from build123d import *

# Parameters (mm, degrees)
SKETCH1_W                                    = 150
SKETCH1_H                                    = 100
EXTRUDE1_DEPTH                               = 20
EXTRUDE2_DEPTH                               = 15
FILLET1_R                                    = 20
CBORE_FOR_M8_HEX_SOCKET_HEAD_CAP_SCR_2_COUNT = 2
CBORE_FOR_M8_HEX_SOCKET_HEAD_CAP_SCR_2_PITCH = 125.099960032
M8_TAPPED_HOLE1_AT_2_COUNT                   = 2
M8_TAPPED_HOLE1_AT_2_PITCH                   = 45
F_8_0_8_DIAMETER_HOLE1_AT_2_COUNT            = 2
F_8_0_8_DIAMETER_HOLE1_AT_2_PITCH            = 70
EXTRUDE3_DEPTH                               = 7
FILLET2_R                                    = 3
FILLET3_R                                    = 10
CHAMFER1_SIZE                                = 0.5
CHAMFER2_SIZE                                = 2
FILLET4_R                                    = 1
SKETCH10_W                                   = 30
SKETCH10_H                                   = 32
EXTRUDE4_DEPTH                               = 5
FILLET5_R                                    = 10
FILLET6_R                                    = 5
SKETCH11_R                                   = 5
EXTRUDE5_DEPTH                               = 1


with BuildPart() as part:
    # Sketch1 → Extrude1 (new body)
    with BuildSketch(Plane.XY):
        with Locations((25, 0)):
            Rectangle(SKETCH1_W, SKETCH1_H)
    extrude(amount=EXTRUDE1_DEPTH)

    # Sketch2 → Extrude2 (add)
    with BuildSketch(Plane.XY.offset(20)):
        with BuildLine():
            Line((60, -15), (60, -30))
            Line((60, -30), (-35, -30))
            Line((-35, -30), (-35, 30))
            Line((-35, 30), (60, 30))
            Line((60, 30), (60, 15))
            ThreePointArc((60, 15), (45, 0), (60, -15))
        make_face()
    extrude(amount=EXTRUDE2_DEPTH)

    # Fillet1
    fillet1_edges = [part.edges().sort_by_distance(p)[0] for p in [
        (-35, 30, 27.5),
        (-35, -30, 27.5),
    ]]
    fillet(fillet1_edges, radius=FILLET1_R)

    # Sketch4 → CBORE for M8 Hex Socket Head Cap Screw1 (revolve, cut)
    with BuildSketch(Plane(origin=(-40, -35, 20), x_dir=(0, -1, 0), z_dir=(1, 0, 0))):
        Polygon((0, 0), (0, 20), (4.5, 20), (4.5, 8.525), (4.525, 8.5), (7.5, 8.5), (7.5, 0), align=None)
    cbore_for_m8_hex_socket_head_cap_screw1 = revolve(axis=Axis((-40, -35, 26.35), (0, 0, -1)), mode=Mode.SUBTRACT)

    # CBORE for M8 Hex Socket Head Cap Scr 2: CBORE for M8 Hex Socket Head Cap Screw1 ×2
    with Locations(*[Vector(0.9992009587217895, 0.03996803834887156, 0) * (i * CBORE_FOR_M8_HEX_SOCKET_HEAD_CAP_SCR_2_PITCH) for i in range(1, CBORE_FOR_M8_HEX_SOCKET_HEAD_CAP_SCR_2_COUNT)]):
        add(cbore_for_m8_hex_socket_head_cap_screw1, mode=Mode.SUBTRACT)

    # Sketch7 → M8 Tapped Hole1 (revolve, cut)
    with BuildSketch(Plane(origin=(-7.5, -20, 35), x_dir=(0, -1, 0), z_dir=(1, 0, 0))):
        Polygon((0, 0), (0, 24.292926105), (3.4, 22.25), (3.4, 0.85), (4.25, 0), align=None)
    m8_tapped_hole1 = revolve(axis=Axis((-7.5, -20, 41.35), (0, 0, -1)), mode=Mode.SUBTRACT)

    # M8 Tapped Hole1 at 2: M8 Tapped Hole1 ×2
    with Locations(*[(i * M8_TAPPED_HOLE1_AT_2_PITCH, 0, 0) for i in range(1, M8_TAPPED_HOLE1_AT_2_COUNT)]):
        add(m8_tapped_hole1, mode=Mode.SUBTRACT)

    # Sketch8 → Ø8.0 (8) Diameter Hole1 (revolve, cut)
    with BuildSketch(Plane(origin=(-20, -22, 35), x_dir=(0, -1, 0), z_dir=(1, 0, 0))):
        Polygon((0, 0), (0, 22.403442476), (4, 20), (4, 0.1), (4.1, 0), align=None)
    f_8_0_8_diameter_hole1 = revolve(axis=Axis((-20, -22, 41.35), (0, 0, -1)), mode=Mode.SUBTRACT)

    # Ø8.0 (8) Diameter Hole1 at 2: Ø8.0 (8) Diameter Hole1 ×2
    with Locations(*[(i * F_8_0_8_DIAMETER_HOLE1_AT_2_PITCH, 0, 0) for i in range(1, F_8_0_8_DIAMETER_HOLE1_AT_2_COUNT)]):
        add(f_8_0_8_diameter_hole1, mode=Mode.SUBTRACT)

    # Mirror1: CBORE for M8 Hex Socket Head Cap Screw1, M8 Tapped Hole1, Ø8.0 (8) Diameter Hole1 across plane
    add(cbore_for_m8_hex_socket_head_cap_screw1.mirror(Plane.ZX), mode=Mode.SUBTRACT)
    add(m8_tapped_hole1.mirror(Plane.ZX), mode=Mode.SUBTRACT)
    add(f_8_0_8_diameter_hole1.mirror(Plane.ZX), mode=Mode.SUBTRACT)

    # Mirror1 copy 1 sketch → Mirror1 copy 1 (revolve, cut)
    with BuildSketch(Plane(origin=(85, 30, 20), x_dir=(0, 1, 0), z_dir=(1, 0, 0))):
        Polygon((0, 0), (0, -20), (4.5, -20), (4.5, -8.525), (4.525, -8.5), (7.5, -8.5), (7.5, 0), align=None)
    revolve(axis=Axis((85, 30, 26.35), (0, 0, 1)), mode=Mode.SUBTRACT)

    # Mirror1 copy 2 sketch → Mirror1 copy 2 (revolve, cut)
    with BuildSketch(Plane(origin=(37.5, 20, 35), x_dir=(0, 1, 0), z_dir=(1, 0, 0))):
        Polygon((0, 0), (0, -24.292926105), (3.4, -22.25), (3.4, -0.85), (4.25, 0), align=None)
    revolve(axis=Axis((37.5, 20, 41.35), (0, 0, 1)), mode=Mode.SUBTRACT)

    # Mirror1 copy 3 sketch → Mirror1 copy 3 (revolve, cut)
    with BuildSketch(Plane(origin=(50, 22, 35), x_dir=(0, 1, 0), z_dir=(1, 0, 0))):
        Polygon((0, 0), (0, -22.403442476), (4, -20), (4, -0.1), (4.1, 0), align=None)
    revolve(axis=Axis((50, 22, 41.35), (0, 0, 1)), mode=Mode.SUBTRACT)

    # Sketch9 → Extrude3 (cut)
    with BuildSketch(Plane.XY.offset(35)):
        with BuildLine():
            Line((21.553843619, 20), (35.695979243, 5.857864376))
            ThreePointArc((35.695979243, 5.857864376), (35, 0), (35.695979243, -5.857864376))
            Line((35.695979243, -5.857864376), (21.553843619, -20))
            Line((21.553843619, -20), (5.267949192, -20))
            Line((5.267949192, -20), (-17, -7.143593539))
            ThreePointArc((-17, -7.143593539), (-20.858895278, -5.545186779), (-25, -5))
            Line((-25, -5), (-25, 5))
            ThreePointArc((-25, 5), (-20.858895278, 5.545186779), (-17, 7.143593539))
            Line((-17, 7.143593539), (5.267949192, 20))
            Line((5.267949192, 20), (21.553843619, 20))
        make_face()
    extrude(amount=-EXTRUDE3_DEPTH, mode=Mode.SUBTRACT)

    # Fillet2
    fillet2_edges = [part.edges().sort_by_distance(p)[0] for p in [
        (-25, -5, 31.5),
        (-25, 5, 31.5),
        (35.695979243, 5.857864376, 31.5),
        (35.695979243, -5.857864376, 31.5),
    ]]
    fillet(fillet2_edges, radius=FILLET2_R)

    # Fillet3
    fillet3_edges = [part.edges().sort_by_distance(p)[0] for p in [
        (5.267949192, 20, 31.5),
        (21.553843619, 20, 31.5),
        (21.553843619, -20, 31.5),
        (5.267949192, -20, 31.5),
    ]]
    fillet(fillet3_edges, radius=FILLET3_R)

    # Chamfer1
    chamfer1_edges = [part.edges().sort_by_distance(p)[0] for p in [
        (-50, 50, 10),
        (100, 50, 10),
        (100, -50, 10),
        (-50, -50, 10),
    ]]
    chamfer(chamfer1_edges, length=CHAMFER1_SIZE)

    # Chamfer2
    chamfer2_edges = [part.edges().sort_by_distance(p)[0] for p in [
        (60, -30, 27.5),
        (60, 30, 27.5),
    ]]
    chamfer(chamfer2_edges, length=CHAMFER2_SIZE)

    # Fillet4
    fillet4_edges = [part.edges().sort_by_distance(p)[0] for p in [
        (60, -15, 27.5),
        (60, 15, 27.5),
    ]]
    fillet(fillet4_edges, radius=FILLET4_R)

    # Sketch10 → Extrude4 (cut)
    with BuildSketch(Plane.XY.offset(20)):
        with Locations((85, 4)):
            Rectangle(SKETCH10_W, SKETCH10_H)
    extrude(amount=-EXTRUDE4_DEPTH, mode=Mode.SUBTRACT)

    # Fillet5
    fillet5_edges = [part.edges().sort_by_distance(p)[0] for p in [
        (70, 20, 17.5),
    ]]
    fillet(fillet5_edges, radius=FILLET5_R)

    # Fillet6
    fillet6_edges = [part.edges().sort_by_distance(p)[0] for p in [
        (70, -12, 17.5),
    ]]
    fillet(fillet6_edges, radius=FILLET6_R)

    # Sketch11 → Extrude5 (cut)
    with BuildSketch(Plane(origin=(0, 0, 0), x_dir=(-1, 0, 0), z_dir=(0, 0, -1))):
        with Locations((40, -35)):
            Circle(SKETCH11_R)
        with Locations((-85, -30)):
            Circle(SKETCH11_R)
        with Locations((-85, 30)):
            Circle(SKETCH11_R)
        with Locations((40, 35)):
            Circle(SKETCH11_R)
    extrude(amount=-EXTRUDE5_DEPTH, mode=Mode.SUBTRACT)


solid = part.part
Here's how the part is built. I have some questions about the finished solid (model axes, mm). A direction names the side the tool comes from. Round coordinates to 2 decimals unless told otherwise and drop trailing zeros. Loops run counter-clockwise (first coordinate to the right, second up) from the corner with the lowest first, then second, coordinate; pieces in that order, holes last. Notation, with made-up numbers: (1.25, 61) - (8.25, 61) arc R22 cw to (8.25, 69) - close; hole circle Ø3 at (33.25, -25.5). An arc over 180 degrees is marked (long way). One line per question, with ' | ' between items. Start each with the question number.
Q1. I want a section at A-A (z = 17.5). State how many separate pieces and enclosed holes the cut face has, then the cut area to 3 significant figures.
Q2. We'd pull the mould along X, two halves only. Please class faces 4 (the cylindrical face through (80.54, -29.41, 6.31)), 5 (the flat face through (100, -1, 10)), 6 (the flat face through (57, 1, 20)): +X half, -X half, draft (parallel to the pull), parting line (faces both ways), or undercut.
Q3. I want a section at C-C (x = 72). Write out the boundary of the cut face in (y, z), then the cut area to 4 significant figures.
Q4. Will these pins go through, and if not, where does the flat tip stop? pin 1 (7 mm diameter, centred on x = 50, y = -22, fed in from +Z); pin 2 (4.5 mm diameter, centred on y = 2, z = 25.5, fed in from -X); pin 3 (4 mm diameter, centred on x = 48, y = 25, fed in from -Z); pin 4 (4.5 mm diameter, centred on x = -42, y = -33.5, fed in from +Z).
Q5. I want a section at D-D (y = 13). Write out the boundary of the cut face in (x, z), then the cut area to 3 significant figures.
Q6. For faces 1 (the cylindrical face through (-28.986, 24.297, 27.605)), 2 (the flat face through (-6.89, -12.98, 31.55)), 3 (the cylindrical face through (-35.005, -34.78, 0.493)), which set-ups out of +Z, -Z, +X, -X, +Y, -Y let a thin tool reach every point of the face, with its end or its side?
Q7. Please list where these lines run through material, in increasing order: line 1 (Y direction, x = -40, z = 17.25); line 2 (Y direction, x = -7.5, z = 27); line 3 (X direction, y = -22, z = 25). Write a range as [from, to].
Response values:
1) separate pieces: 1 | enclosed holes: 12 | area: 13,000 mm²
2) face 4: undercut | face 5: +X half | face 6: draft
3) outline: (-50, 0) - (50, 0) - (50, 20) - (16, 20) - (16, 15) - (-11, 15) - (-11, 20) - (-50, 20) - close | area: 1,865 mm²
4) pin 1: stops at z = 14.7 | pin 2: stops at x = -35 | pin 3: stops at z = 0 | pin 4: stops at z = 11.5
5) outline: (-50, 0) - (100, 0) - (100, 15) - (70.46, 15) - (70.46, 20) - (52.52, 20) - (52.52, 35) - (28.55, 35) - (28.55, 28) - (-6.86, 28) - (-6.86, 35) - (-34.77, 35) - (-34.77, 20) - (-50, 20) - close | area: 3,910 mm²
6) face 1: +Z, -X, +Y | face 2: +Z | face 3: -Z
7) line 1: y = [-50, -42.5], [-27.5, 27.5], [42.5, 50] | line 2: y = [-30, -23.4], [-16.6, 16.6], [23.4, 30] | line 3: x = [-31, -24], [-16, -10.25], [-4.75, 34.75], [40.25, 46], [54, 60]
